Verification items for this drawing (mm, ordinates from the low corner). A direction names the side the tool comes from. Give positions to 0.01 mm unless a question says otherwise; leave off trailing zeros. Loops run counter-clockwise (first coordinate to the right, second up) from the corner with the lowest first, then second, coordinate; pieces in that order, holes last. Notation, with made-up numbers: (89.25, 53.5) -> (100.25, 53.5) arc R27 ccw to (100.25, 73.5) -> close; hole circle Ø9 at (77, -17). An arc over 180 degrees is marked (long way). Answer in a Markdown table with one row per item. Add a question column.
Q1. Section check D-D on y = 33. Enter the section's corners in (x, z).
Q2. Release check for a two-part mould opening along Y. For the marked faces 1, 2 and 3 record: pulls with the +Y half, pulls with the -Y half, needs draft (parallel to the pull), parting line crosses it, or undercut.
Q3. Material ranges on probe 1 along Z at (x, y) = (13.75, 25); probe 2 along Z at (x, y) = (6, 25); probe 3 along X at (y, z) = (22, 21.5), recorded low to high.
Q4. Section check C-C on x = 54. Enter the section's corners in (y, z).
Q5. Section check A-A on z = 56. Enter the section's corners in (x, y), and give its area (3 significant figures).
Q6. Set-up check for the marked faces 4, 5, 6, 7 and 8: record each of +Z, -Z, +X, -X, +Y, -Y from which the full face is reachable in a straight line by a thin tool's end or side.
Q7. Section check B-B on x = 13.5. Enter the section's corners in (y, z).
Q8. Gauge pin test, flat ends, axial feed: P1, Ø2, axis at y = 37, z = 71.5, coming from the +X side; P2, Ø2, axis at x = 22.5, z = 41.5, coming from the -Y side; P3, Ø6, axis at x = 19.5, y = 30.5, coming from the +Z side. Record the tip position at first contact, or that the pin passes through.
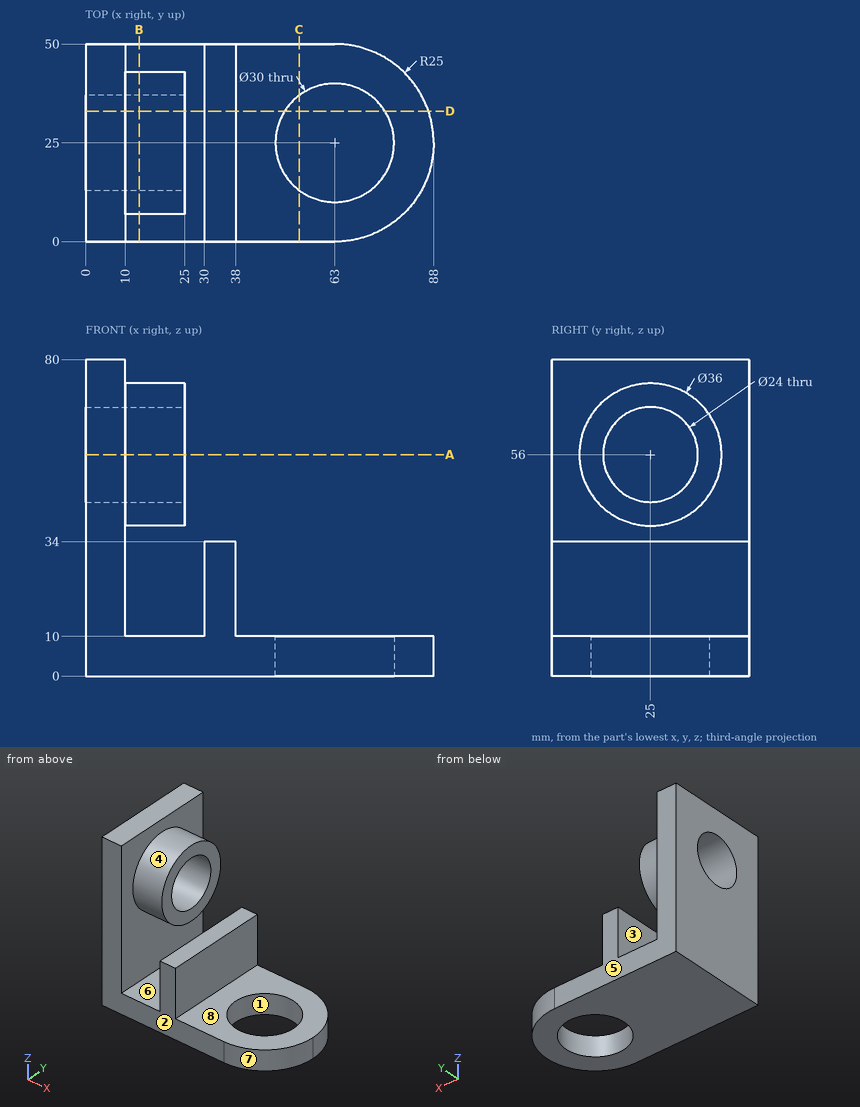
Taken from the geometry:
| question | item | result |
|---|---|---|
| 1 | outline | (0, 0) -> (50.31, 0) -> (50.31, 10) -> (38, 10) -> (38, 34) -> (30, 34) -> (30, 10) -> (10, 10) -> (10, 39.88) -> (25, 39.88) -> (25, 47.06) -> (0, 47.06) -> close; (0, 64.94) -> (25, 64.94) -> (25, 72.12) -> (10, 72.12) -> (10, 80) -> (0, 80) -> close; (75.69, 0) -> (86.69, 0) -> (86.69, 10) -> (75.69, 10) -> close |
| 2 | face 1 | undercut |
| 2 | face 2 | pulls with the -Y half |
| 2 | face 3 | needs draft |
| 3 | probe 1 | z = 0 to 10, 38 to 44, 68 to 74 |
| 3 | probe 2 | z = 0 to 44, 68 to 80 |
| 3 | probe 3 | x = 0 to 10, 30 to 38 |
| 4 | outline | (0, 0) -> (13, 0) -> (13, 10) -> (0, 10) -> close; (37, 0) -> (50, 0) -> (50, 10) -> (37, 10) -> close |
| 5 | outline | (0, 0) -> (10, 0) -> (10, 7) -> (25, 7) -> (25, 13) -> (0, 13) -> close; (0, 37) -> (25, 37) -> (25, 43) -> (10, 43) -> (10, 50) -> (0, 50) -> close |
| 5 | area | 440 mm² |
| 6 | face 4 | +X |
| 6 | face 5 | +Z, -Z, +X, -X, +Y |
| 6 | face 6 | +Y, -Y |
| 6 | face 7 | +Z, -Z, +X, -Y |
| 6 | face 8 | +Z, +X, +Y, -Y |
| 7 | outline | (0, 0) -> (50, 0) -> (50, 10) -> (0, 10) -> close; circle Ø36 at (25, 56); hole circle Ø24 at (25, 56) |
| 8 | P1 | stops at x = 10 |
| 8 | P2 | stops at y = 13.09 |
| 8 | P3 | stops at z = 73.83 |
